Geometry check sheet. Reference: drawing and pictorial views, mm from the part's lowest x, y, z. A direction names the side the tool comes from. Give positions to 0.01 mm unless a question says otherwise; leave off trailing zeros. Order: outer loops, then holes, each group sorted by start corner. A loop starts at its lowest first (then second) coordinate and runs counter-clockwise, first axis right, second up. Notation, with made-up numbers: (81, 31) - (132, 31) arc R22 ccw to (132, 67) - close; hole circle Ø8 at (52.25, 27). An arc over 180 degrees is marked (long way). Answer as a JSON object with one key per item and string values.
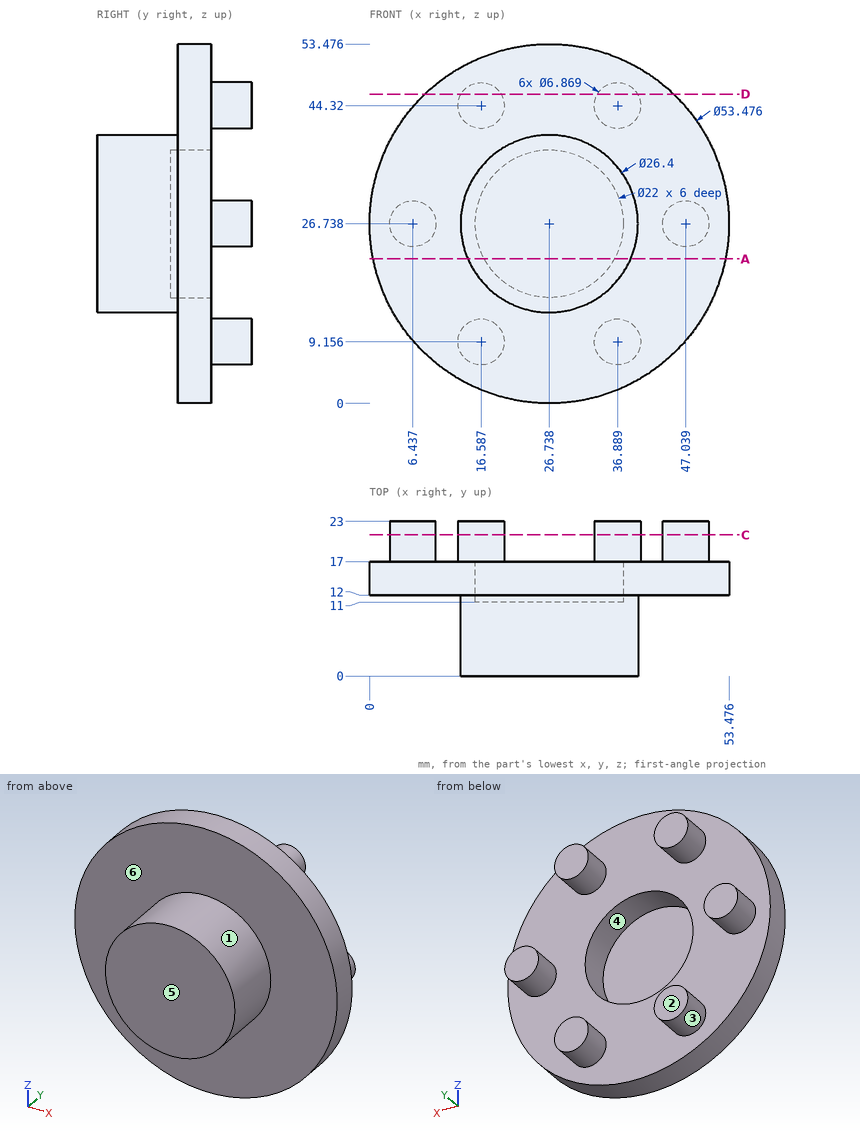
(1) Access from +Z, -Z, +X, -X, +Y, -Y to the whole of each face (thin tool, end or side, straight path). Record for the marked faces 4, 5 and 6.
Computed values:
{"face 4": "+Y", "face 5": "+Z, -Z, +X, -X, -Y", "face 6": "-Y"}
(2) Material ranges on line 1 along Z through (x, y) = (26.5, 14.5) (1 decimal); line 2 along Y through (x, z) = (25.5, 15.5); line 3 along Y through (x, z) = (33, 21), recorded low to high. Write a range as [from, to].
Computed values:
{"line 1": "z = [0, 15.7], [37.7, 53.5]", "line 2": "y = [0, 17]", "line 3": "y = [0, 11]"}
(3) Section check D-D (z = 46). Record the cut outline in (x, y), then the cut area to 3 significant figures.
Computed values:
{"outline": "(8.19, 12) - (45.28, 12) - (45.28, 17) - (39.88, 17) - (39.88, 23) - (33.89, 23) - (33.89, 17) - (19.58, 17) - (19.58, 23) - (13.59, 23) - (13.59, 17) - (8.19, 17) - close", "area": "257 mm²"}
(4) Section check A-A (z = 21.5). Record the cut outline in (x, y) (1 decimal).
Computed values:
{"outline": "(0.5, 12) - (14.6, 12) - (14.6, 0) - (38.9, 0) - (38.9, 12) - (53, 12) - (53, 17) - (36.4, 17) - (36.4, 11) - (17.1, 11) - (17.1, 17) - (0.5, 17) - close"}
(5) Release check for a two-part mould opening along Z. For the marked faces 1, 2 and 3 record: pulls with the +Z half, pulls with the -Z half, needs draft (parallel to the pull), parting line crosses it, or undercut.
Computed values:
{"face 1": "parting line crosses it", "face 2": "needs draft", "face 3": "undercut"}
(6) Gauge pin test, flat ends, axial feed: pin 1 Ø2 at (x, y) = (22.5, 14) entering from +Z; pin 2 Ø10 at (x, y) = (19, 15) entering from -Z; pin 3 Ø6 at (y, z) = (14.5, 7) entering from -X. Record the tip position at first contact, or that the pin passes through.
Computed values:
{"pin 1": "stops at z = 53.28", "pin 2": "stops at z = 0.14", "pin 3": "stops at x = 5.89"}
(7) Section check C-C (y = 21). Record the cut outline in (x, z) (1 decimal), then the cut area to 3 significant figures.
Computed values:
{"outline": "circle Ø6.9 at (6.4, 26.7); circle Ø6.9 at (16.6, 9.2); circle Ø6.9 at (16.6, 44.3); circle Ø6.9 at (36.9, 9.2); circle Ø6.9 at (36.9, 44.3); circle Ø6.9 at (47, 26.7)", "area": "222 mm²"}
